```python
from build123d import *

# Parameters (mm, degrees)
SKETCH_1_R             = 3
EXTRUDE_1_DEPTH        = 12
SKETCH_2_R             = 1.4
EXTRUDE_2_DEPTH        = 3
CHAMFER_1_SIZE         = 0.5
HOLE_WIZARD_M3_1_D     = 2.5
HOLE_WIZARD_M3_1_DEPTH = 7.5
HOLE_WIZARD_M3_1_TIP   = 0.751075774
SKETCH_7_W             = 9.702446008
SKETCH_7_H             = 5
CUT_EXTRUDE_1_DEPTH    = 0.5


with BuildPart() as part:
    # 草图1 → 凸台-拉伸1 (new body)
    with BuildSketch(Plane.XY):
        Circle(SKETCH_1_R)
    extrude(amount=EXTRUDE_1_DEPTH)

    # 草图2 → 凸台-拉伸2 (add)
    with BuildSketch(Plane.XY.offset(12)):
        Circle(SKETCH_2_R)
    extrude(amount=EXTRUDE_2_DEPTH)

    # 倒角1
    chamfer_1_edges = [part.edges().sort_by_distance(p)[0] for p in [
        (-3, 0, 0),
        (-3, 0, 12),
        (-1.4, 0, 15),
    ]]
    chamfer(chamfer_1_edges, length=CHAMFER_1_SIZE)

    # M3 螺纹孔1
    with Locations(Plane(origin=(0, 0, 0), x_dir=(-1, 0, 0), z_dir=(0, 0, -1))):
        with Locations((0, 0)):
            Hole(HOLE_WIZARD_M3_1_D / 2, depth=HOLE_WIZARD_M3_1_DEPTH)
            with Locations((0, 0, -(HOLE_WIZARD_M3_1_DEPTH + HOLE_WIZARD_M3_1_TIP / 2))):  # 118° drill point
                Cone(0, HOLE_WIZARD_M3_1_D / 2, HOLE_WIZARD_M3_1_TIP, mode=Mode.SUBTRACT)

    # 草图7 → 切除-拉伸1 (cut)
    with BuildSketch(Plane(origin=(0, 3, 0), x_dir=(-1, 0, 0), z_dir=(0, 1, 0))):
        with Locations((0, 8.5)):
            Rectangle(SKETCH_7_W, SKETCH_7_H)
    cut_extrude_1 = extrude(amount=-CUT_EXTRUDE_1_DEPTH, mode=Mode.SUBTRACT)

    # 镜向1: 切除-拉伸1 across plane
    add(cut_extrude_1.mirror(Plane.ZX), mode=Mode.SUBTRACT)


solid = part.part
```
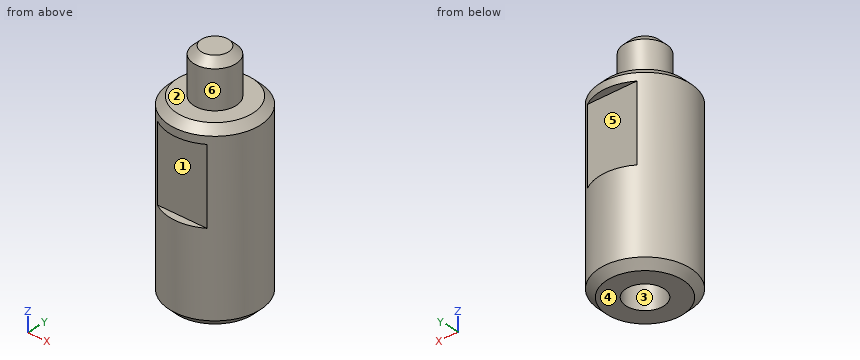
The listing builds one solid part. Answer for the finished solid, in the listing's coordinates (mm). Face numbers are marked on the shaded views. A direction names the side the tool comes from. Round coordinates to 2 decimals unless told otherwise and drop trailing zeros. Write each loop counter-clockwise with the first axis right and the second up, starting at its lowest first coordinate (ties: lowest second). Pieces come first, ordered by that corner, then holes. Notation, with made-up numbers: (75.5, 66.25) -> (99.5, 66.25) arc R20 cw to (99.5, 83.25) -> close; hole circle Ø11 at (34, -1.75). An arc over 180 degrees is marked (long way). Answer as a JSON object with one key per item and string values. Group by question number.
Q1. Straight lines are drawn through the part: line 1 along Y through (x, z) = (0, 4.75); line 2 along X through (y, z) = (0.1, 12.5); line 3 along Z through (x, y) = (2.05, 0.95). For each, find the intervals that lie inside material, in ascending order.
Q2. Each of these flat-tipped pins is pushed along its axis until it touches: pin 1 Ø3.5 at (x, z) = (0, 8) entering from +Y; pin 2 Ø1.7 at (x, z) = (0, 8) entering from -Y; pin 3 Ø1 at (x, z) = (1, 11.5) entering from +Y; pin 4 Ø2 at (x, y) = (1, -1) entering from +Z. Where does it stop, or does it pass through?
Q3. Determine the mould class of the marked faces 1, 2 and 3 for opening direction Z: pulls with the +Z half, pulls with the -Z half, needs draft (parallel to the pull), parting line crosses it, or undercut.
Q4. Section A-A (z = 3.75) is taken. Write down the section's boundary in (x, y), plus the area to 3 significant figures.
Q5. Which of the six approach directions +Z, -Z, +X, -X, +Y, -Y give full straight-line access (tool end or side, diameter ignored) to the marked faces 4, 5 and 6?
Check values:
{
 "1": {"line 1": "-3 to -1.25, 1.25 to 3", "line 2": "-1.4 to 1.4", "line 3": "0 to 12"},
 "2": {"pin 1": "y = 2.5", "pin 2": "y = -2.5", "pin 3": "y = 2.96", "pin 4": "z = 15"},
 "3": {"face 1": "undercut", "face 2": "pulls with the +Z half", "face 3": "needs draft"},
 "4": {"outline": "circle Ø6 at (0, 0); hole circle Ø2.5 at (0, 0)", "area": "23.4 mm^2"},
 "5": {"face 4": "-Z, +X, -X, +Y, -Y", "face 5": "+X, -X, +Y", "face 6": "+Z"}
}
